Geometry: final body of the model. Coordinates: model frame, mm. A direction names the side the tool comes from. Give positions to 0.01 mm unless a question says otherwise; leave off trailing zeros. Write each loop counter-clockwise with the first axis right and the second up, starting at its lowest first coordinate (ties: lowest second). Pieces come first, ordered by that corner, then holes. Notation, with made-up numbers: M 24.5,-32.75 L 68.5,-32.75 A31 ccw 68.5,-3.75 Z; hole C 59,-37.5 d5. An arc over 180 degrees is marked long. Use one line per item in the form item = value. Start each with the question number.
Item 1: Material intervals for line 1 along X through (y, z) = (2.75, 0); line 2 along Z through (x, y) = (0, 5); line 3 along X through (y, z) = (2.75, 4.5), sorted ascending. Write a range as from..to.
Item 2: Contact query for flat-ended pins moving along their axis: P1, Ø1.5, axis at x = 4.5, y = 4, coming from the +Z side; P2, Ø3, axis at x = -4, y = 5.5, coming from the -Z side; P3, Ø1.5, axis at x = -4.5, z = 6, coming from the -Y side; P4, Ø3, axis at x = 2.5, z = -4, coming from the -Y side. Output: stop coordinate, or through.
Item 3: Section query B-B on y = 5. Return loops of the section in (x, z), then the cut area to 3 significant figures.
Item 4: Access query for faces 5 (the cylindrical face through (0, 5, -7)), 6 (the flat face through (2, 5, 13)), 7 (the flat face through (-2, 5, 13)). Directions: +Z, -Z, +X, -X, +Y, -Y. A direction counts if a zero-diameter tool reaches every point of the face in a straight line with its end or side. Return the directions, or none.
Item 5: Section query D-D on y = 1. Return loops of the section in (x, z).
Item 6: Section query A-A on z = 6. Return loops of the section in (x, y).
Item 7: Pull-direction query (X, two-part tool) for faces 1 (the flat face through (0, 0, 7)), 2 (the cylindrical face through (5.96, 4.93, -1.88)), 3 (the flat face through (-7, 5, 4)), 4 (the flat face through (7, 5, 4)); classes: released by +X, released by -X, zero draft, split by the parting line, or undercut.
Item 8: Section query C-C on x = -1.75. Return loops of the section in (y, z).
from build123d import *

# Parameters (mm, degrees)
SKETCH1_R                = 7
SKETCH1_R_2              = 6.25
BOSS_EXTRUDE1_DEPTH      = 10
SKETCH3_W                = 14
SKETCH3_H                = 10
BOSS_EXTRUDE2_DEPTH      = 8
SKETCH4_R                = 6.25
CUT_EXTRUDE1_DEPTH       = 20
BOSS_EXTRUDE3_DEPTH      = 2
BOSS_EXTRUDE3_DEPTH_BACK = 2


with BuildPart() as part:
    # Sketch1 → Boss-Extrude1 (new body)
    with BuildSketch(Plane(origin=(0, 0, 0), x_dir=(1, 0, 0), z_dir=(0, 1, 0))):
        Circle(SKETCH1_R)
        Circle(SKETCH1_R_2, mode=Mode.SUBTRACT)
    extrude(amount=BOSS_EXTRUDE1_DEPTH)

    # Sketch3 → Boss-Extrude2 (add)
    with BuildSketch(Plane.XY):
        with Locations((0, 5)):
            Rectangle(SKETCH3_W, SKETCH3_H)
    extrude(amount=BOSS_EXTRUDE2_DEPTH)

    # Sketch4 → Cut-Extrude1 (cut)
    with BuildSketch(Plane(origin=(0, 10, 0), x_dir=(1, 0, 0), z_dir=(0, 1, 0))):
        Circle(SKETCH4_R)
    extrude(amount=-CUT_EXTRUDE1_DEPTH, mode=Mode.SUBTRACT)

    # Sketch6 → Boss-Extrude3 (add, two sides)
    with BuildSketch(Plane(origin=(0, 0, 0), x_dir=(0, 0, -1), z_dir=(1, 0, 0))) as boss_extrude3_sk:
        with BuildLine():
            Line((-8, 10), (-13, 10))
            ThreePointArc((-13, 10), (-18, 5), (-13, 0))
            Line((-13, 0), (-8, 0))
            Line((-8, 0), (-8, 10))
        make_face()
    extrude(amount=BOSS_EXTRUDE3_DEPTH)
    extrude(boss_extrude3_sk.sketch, amount=-BOSS_EXTRUDE3_DEPTH_BACK)


solid = part.part
Answer sheet:
q1.line_1 = -7..-6.25, 6.25..7
q1.line_2 = -7..-6.25, 6.25..18
q1.line_3 = -7..-4.34, 4.34..7
q2.P1 = 8
q2.P2 = -6.54
q2.P3 = 0
q2.P4 = through
q3.outline = M -7,0 A7 ccw 7,0 L 7,8 L 2,8 L 2,18 L -2,18 L -2,8 L -7,8 Z; hole C 0,0 d12.5
q3.area = 106 mm2
q4.face_5 = -Z, +Y, -Y
q4.face_6 = +Z, +X, +Y, -Y
q4.face_7 = +Z, -X, +Y, -Y
q5.outline = M -7,0 A7 ccw 7,0 L 7,8 L 2,8 L 2,16 L -2,16 L -2,8 L -7,8 Z; hole C 0,0 d12.5
q6.outline = M -7,0 L -1.75,0 L -1.75,10 L -7,10 Z; M 1.75,0 L 7,0 L 7,10 L 1.75,10 Z
q7.face_1 = zero draft
q7.face_2 = undercut
q7.face_3 = released by -X
q7.face_4 = released by +X
q8.outline = M 0,-6.78 L 10,-6.78 L 10,-6 L 0,-6 Z; M 0,6 L 10,6 L 10,13 A5 ccw 0,13 Z
